from build123d import *

# Parameters (mm, degrees)
SKETCH1_W             = 15.5
SKETCH1_H             = 45
BOSS_EXTRUDE1_DEPTH   = 5
BOSS_EXTRUDE1_2_DEPTH = 5
SKETCH1_R             = 2.6
BOSS_EXTRUDE1_3_DEPTH = 5
BOSS_EXTRUDE1_4_DEPTH = 5
SKETCH1_3_W           = 1
SKETCH1_3_H           = 45
BOSS_EXTRUDE2_DEPTH   = 5.2
SKETCH1_4_W           = 5
SKETCH1_4_H           = 45
SKETCH1_4_W_2         = 10
SKETCH1_4_R           = 2.6
BOSS_EXTRUDE3_DEPTH   = 7
SKETCH2_W             = 7.5
SKETCH2_H             = 15
CUT_EXTRUDE1_DEPTH    = 1.1
SKETCH3_R             = 3.1
CUT_EXTRUDE2_DEPTH    = 152.506600516
SKETCH5_W             = 20
SKETCH5_H             = 20
SKETCH5_W_2           = 14.9
SKETCH5_H_2           = 14.9
BOSS_EXTRUDE4_DEPTH   = 3
SKETCH5_3_W           = 14.9
SKETCH5_3_H           = 14.9
BOSS_EXTRUDE5_DEPTH   = 4.9
BOSS_EXTRUDE6_START   = 7
SKETCH5_4_W           = 20
SKETCH5_4_H           = 20
SKETCH5_4_W_2         = 15.2
SKETCH5_4_H_2         = 15.2
BOSS_EXTRUDE6_DEPTH   = 3.9
BOSS_EXTRUDE7_START   = 7
SKETCH5_5_W           = 15.2
SKETCH5_5_H           = 15.2
BOSS_EXTRUDE7_DEPTH   = 1
FILLET1_R             = 2
BOSS_EXTRUDE8_START   = -7
SKETCH6_W             = 10
SKETCH6_H             = 10
BOSS_EXTRUDE8_DEPTH   = 3
CHAMFER1_SIZE         = 1
SKETCH8_W             = 20
SKETCH8_H             = 15
SKETCH8_W_2           = 10.7
SKETCH8_H_2           = 10.15
BOSS_EXTRUDE9_DEPTH   = 3
SKETCH8_3_W           = 4
SKETCH8_3_H           = 10.15
BOSS_EXTRUDE10_DEPTH  = 0.6
FILLET3_R             = 2


with BuildPart() as part:
    # Sketch1 → Boss-Extrude1 (new body)
    with BuildSketch(Plane(origin=(0, 0, 0), x_dir=(1, 0, 0), z_dir=(0, 1, 0))):
        with Locations((73.25, 22.5)):
            Rectangle(SKETCH1_W, SKETCH1_H)
    extrude(amount=BOSS_EXTRUDE1_DEPTH)



with BuildPart() as body_2:
    # Sketch1 → Boss-Extrude1 2 (new body)
    with BuildSketch(Plane(origin=(0, 0, 0), x_dir=(1, 0, 0), z_dir=(0, 1, 0))):
        with Locations((89.75, 22.5)):
            Rectangle(SKETCH1_W, SKETCH1_H)
    extrude(amount=BOSS_EXTRUDE1_2_DEPTH)


with BuildPart() as body_3:
    # Sketch1 → Boss-Extrude1 3 (new body)
    with BuildSketch(Plane(origin=(0, 0, 0), x_dir=(1, 0, 0), z_dir=(0, 1, 0))):
        with Locations((110.25, 22.5)):
            Rectangle(SKETCH1_W, SKETCH1_H)
        with Locations(Location((110.25, 20, 0), (0, 0, 270))):
            Circle(SKETCH1_R, mode=Mode.SUBTRACT)
        with Locations(Location((110.25, 27.5, 0), (0, 0, 270))):
            Circle(SKETCH1_R, mode=Mode.SUBTRACT)
        with Locations(Location((110.25, 35, 0), (0, 0, 270))):
            Circle(SKETCH1_R, mode=Mode.SUBTRACT)
    extrude(amount=BOSS_EXTRUDE1_3_DEPTH)


with BuildPart() as body_4:
    # Sketch1 → Boss-Extrude1 4 (new body)
    with BuildSketch(Plane(origin=(0, 0, 0), x_dir=(1, 0, 0), z_dir=(0, 1, 0))):
        with Locations((126.75, 22.5)):
            Rectangle(SKETCH1_W, SKETCH1_H)
        with Locations(Location((126.75, 20, 0), (0, 0, 270))):
            Circle(SKETCH1_R, mode=Mode.SUBTRACT)
        with Locations(Location((126.75, 27.5, 0), (0, 0, 270))):
            Circle(SKETCH1_R, mode=Mode.SUBTRACT)
        with Locations(Location((126.75, 35, 0), (0, 0, 270))):
            Circle(SKETCH1_R, mode=Mode.SUBTRACT)
    extrude(amount=BOSS_EXTRUDE1_4_DEPTH)


with BuildPart() as part_1:
    add(part.part)

    add(body_2.part)  # Boss-Extrude2 merges body 2

    add(body_3.part)  # Boss-Extrude2 merges body 3

    add(body_4.part)  # Boss-Extrude2 merges body 4
    # Sketch1<3> → Boss-Extrude2 (add)
    with BuildSketch(Plane(origin=(0, 0, 0), x_dir=(1, 0, 0), z_dir=(0, 1, 0))):
        with Locations((81.5, 22.5)):
            Rectangle(SKETCH1_3_W, SKETCH1_3_H)
        with Locations((118.5, 22.5)):
            Rectangle(SKETCH1_3_W, SKETCH1_3_H)
    extrude(amount=BOSS_EXTRUDE2_DEPTH)

    # Sketch1<4> → Boss-Extrude3 (add)
    # profile 1 of 3: a face of its own
    with BuildSketch(Plane(origin=(0, 0, 0), x_dir=(1, 0, 0), z_dir=(0, 1, 0))):
        with Locations((100, 22.5)):
            Rectangle(SKETCH1_4_W, SKETCH1_4_H)
    # profile 2 of 3: a face of its own
    with BuildSketch(Plane(origin=(0, 0, 0), x_dir=(1, 0, 0), z_dir=(0, 1, 0))):
        with Locations((139.5, 22.5)):
            Rectangle(SKETCH1_4_W_2, SKETCH1_4_H)
        with Locations(Location((139.5, 31.5, 0), (0, 0, 270))):
            Circle(SKETCH1_4_R, mode=Mode.SUBTRACT)
        with Locations(Location((139.5, 39, 0), (0, 0, 270))):
            Circle(SKETCH1_4_R, mode=Mode.SUBTRACT)
    # profile 3 of 3: a face of its own
    with BuildSketch(Plane(origin=(0, 0, 0), x_dir=(1, 0, 0), z_dir=(0, 1, 0))):
        with Locations((60.5, 22.5)):
            Rectangle(SKETCH1_4_W_2, SKETCH1_4_H)
    extrude(amount=BOSS_EXTRUDE3_DEPTH)

    # Sketch2 → Cut-Extrude1 (cut)
    with BuildSketch(Plane(origin=(0, 0, 0), x_dir=(-1, 0, 0), z_dir=(0, -1, 0))):
        with Locations((-139.5, 35.25)):
            Rectangle(SKETCH2_W, SKETCH2_H)
    extrude(amount=-CUT_EXTRUDE1_DEPTH, mode=Mode.SUBTRACT)

    # Sketch3 → Cut-Extrude2 (cut, through all)
    with BuildSketch(Plane(origin=(0, 7, 0), x_dir=(1, 0, 0), z_dir=(0, 1, 0))):
        with Locations(Location((60.5, 6, 0), (0, 0, 270))):
            Circle(SKETCH3_R)
        with Locations(Location((139.5, 6, 0), (0, 0, 90))):
            Circle(SKETCH3_R)
    extrude(amount=-CUT_EXTRUDE2_DEPTH, mode=Mode.SUBTRACT)

    # Sketch5 → Boss-Extrude4 (add)
    # profile 1 of 2: a face of its own
    with BuildSketch(Plane(origin=(0, 0, 0), x_dir=(1, 0, 0), z_dir=(0, 1, 0))):
        with Locations((154.5, 35)):
            Rectangle(SKETCH5_W, SKETCH5_H)
        with Locations((154.5, 35)):
            Rectangle(SKETCH5_W_2, SKETCH5_H_2, mode=Mode.SUBTRACT)
    # profile 2 of 2: a face of its own
    with BuildSketch(Plane(origin=(0, 0, 0), x_dir=(1, 0, 0), z_dir=(0, 1, 0))):
        with Locations((154.5, 35)):
            Rectangle(SKETCH5_W_2, SKETCH5_H_2)
    extrude(amount=BOSS_EXTRUDE4_DEPTH)

    # Sketch5<3> → Boss-Extrude5 (add)
    with BuildSketch(Plane(origin=(0, 0, 0), x_dir=(1, 0, 0), z_dir=(0, 1, 0))):
        with Locations((154.5, 35)):
            Rectangle(SKETCH5_3_W, SKETCH5_3_H)
    extrude(amount=BOSS_EXTRUDE5_DEPTH)

    # Sketch5<4> → Boss-Extrude6 (add)
    with BuildSketch(Plane(origin=(0, 0, 0), x_dir=(1, 0, 0), z_dir=(0, 1, 0)).offset(BOSS_EXTRUDE6_START)):
        with Locations((45.5, 35)):
            Rectangle(SKETCH5_4_W, SKETCH5_4_H)
        with Locations((45.5, 35)):
            Rectangle(SKETCH5_4_W_2, SKETCH5_4_H_2, mode=Mode.SUBTRACT)
    extrude(amount=-BOSS_EXTRUDE6_DEPTH)

    # Sketch5<5> → Boss-Extrude7 (add)
    with BuildSketch(Plane(origin=(0, 0, 0), x_dir=(1, 0, 0), z_dir=(0, 1, 0)).offset(BOSS_EXTRUDE7_START)):
        with Locations((45.5, 35)):
            Rectangle(SKETCH5_5_W, SKETCH5_5_H)
    extrude(amount=-BOSS_EXTRUDE7_DEPTH)

    # Fillet1
    fillet1_edges = [part_1.edges().sort_by_distance(p)[0] for p in [
        (161.95, 3.95, -42.45),
        (147.05, 3.95, -42.45),
        (147.05, 3.95, -27.55),
        (161.95, 3.95, -27.55),
    ]]
    fillet(fillet1_edges, radius=FILLET1_R)

    # Sketch6 → Boss-Extrude8 (add)
    with BuildSketch(Plane(origin=(0, 7, 0), x_dir=(1, 0, 0), z_dir=(0, 1, 0)).offset(BOSS_EXTRUDE8_START)):
        with Locations((60.5, 50)):
            Rectangle(SKETCH6_W, SKETCH6_H)
    extrude(amount=BOSS_EXTRUDE8_DEPTH)

    # Chamfer1
    chamfer1_edges = [part_1.edges().sort_by_distance(p)[0] for p in [
        (45.5, 3.1, -45),
    ]]
    chamfer(chamfer1_edges, length=CHAMFER1_SIZE)

    # Sketch8 → Boss-Extrude9 (add)
    with BuildSketch(Plane(origin=(0, 0, 0), x_dir=(1, 0, 0), z_dir=(0, 1, 0))):
        with Locations((154.5, 17.5)):
            Rectangle(SKETCH8_W, SKETCH8_H)
        with Locations((154.5, 17.5)):
            Rectangle(SKETCH8_W_2, SKETCH8_H_2, mode=Mode.SUBTRACT)
    extrude(amount=BOSS_EXTRUDE9_DEPTH)

    # Sketch8<3> → Boss-Extrude10 (add)
    with BuildSketch(Plane(origin=(0, 0, 0), x_dir=(1, 0, 0), z_dir=(0, 1, 0))):
        with Locations((154.5, 17.5)):
            Rectangle(SKETCH8_3_W, SKETCH8_3_H)
    extrude(amount=BOSS_EXTRUDE10_DEPTH)

    # Fillet3
    fillet3_edges = [part_1.edges().sort_by_distance(p)[0] for p in [
        (164.5, 1.5, -45),
        (35.5, 5.05, -25),
        (65.5, 1.5, -55),
        (55.5, 1.5, -55),
        (164.5, 1.5, -10),
        (97.5, 6, -45),
        (102.5, 6, -45),
        (134.5, 6, -45),
        (144.5, 3.5, 0),
        (144.5, 5, -45),
        (55.5, 3.5, 0),
        (65.5, 6, -45),
    ]]
    fillet(fillet3_edges, radius=FILLET3_R)


solid = part_1.part
Model file for the job. Use its own axes, mm. A direction names the side the tool comes from. Round coordinates to 2 decimals unless told otherwise and drop trailing zeros. Order: outer loops, then holes, each group sorted by start corner. A loop starts at its lowest first (then second) coordinate and runs counter-clockwise, first axis right, second up. Notation, with made-up numbers: M 38.25,26 L 57.25,26 A20 cw 57.25,33 Z; hole C 56,-34.75 d3. An arc over 180 degrees is marked long. Write each question's results on one line, items separated by ' | '. Start each with the question number.
(1) Probe probe 1 along Z at (x, y) = (139.5, 4.15); probe 2 along X at (y, z) = (6.5, -35); probe 3 along X at (y, z) = (2.75, -27). List the from-to ranges inside material, lowest first. Write a range as from..to.
(2) Saw through at A-A, the plane x = 110.25. Give the cut face in (y, z).
(3) Which spindle directions (+Z, -Z, +X, -X, +Y, -Y) get a long thin tool onto all of the face, cutting with end or side? Do faces 1 (the face through (159.85, 1, -17)), 2 (the face through (60, 3, -50)), 3 (the face through (53.1, 5, -35)). Say none if no direction does.
(4) Drop flat-ended pins along their axis: pin 1 (1 mm diameter, centred on y = 6.5, z = -15, fed in from -X); pin 2 (1.5 mm diameter, centred on x = 104, z = -19, fed in from +Y); pin 3 (0.8 mm diameter, centred on x = 81.5, z = -15.5, fed in from +Y). Give the stop position or say it passes through.
(5) Two-plate mould, pull along Z, no slides. Class faces 4 (the face through (154, 0.6, -18)), 5 (the face through (153, 1, -10)), 6 (the face through (144.5, 4, -18)): pulls with the +Z half, pulls with the -Z half, needs draft (parallel to the pull), parting line crosses it, or undercut.
(6) Saw through at C-C, the plane z = -14.5. State how many separate pieces and enclosed holes the cut face has, then the cut area to 3 significant figures.
(7) Saw through at B-B, the plane x = 60.5. Give the cut face in (y, z).
Established:
1) probe 1: z = -45..-41.6, -36.4..-34.1, -28.9..-9.1, -2.9..0 | probe 2: x = 35.5..65.5, 97.5..102.5, 134.5..144.5 | probe 3: x = 55.5..107.7, 112.8..124.2, 129.3..164.5
2) outline: M 0,-45 L 5,-45 L 5,-37.6 L 0,-37.6 Z; M 0,-32.4 L 5,-32.4 L 5,-30.1 L 0,-30.1 Z; M 0,-24.9 L 5,-24.9 L 5,-22.6 L 0,-22.6 Z; M 0,-17.4 L 5,-17.4 L 5,0 L 0,0 Z
3) face 1: +Y, -Y | face 2: -Z, +X, -X, +Y | face 3: -Y
4) pin 1: stops at x = 55.5 | pin 2: stops at y = 5 | pin 3: stops at y = 5.2
5) face 4: undercut | face 5: pulls with the +Z half | face 6: needs draft
6) separate pieces: 3 | enclosed holes: 0 | area: 526 mm^2
7) outline: M 0,-55 L 3,-55 L 3,-45 L 7,-45 L 7,-9.1 L 0,-9.1 Z; M 0,-2.9 L 7,-2.9 L 7,0 L 0,0 Z
